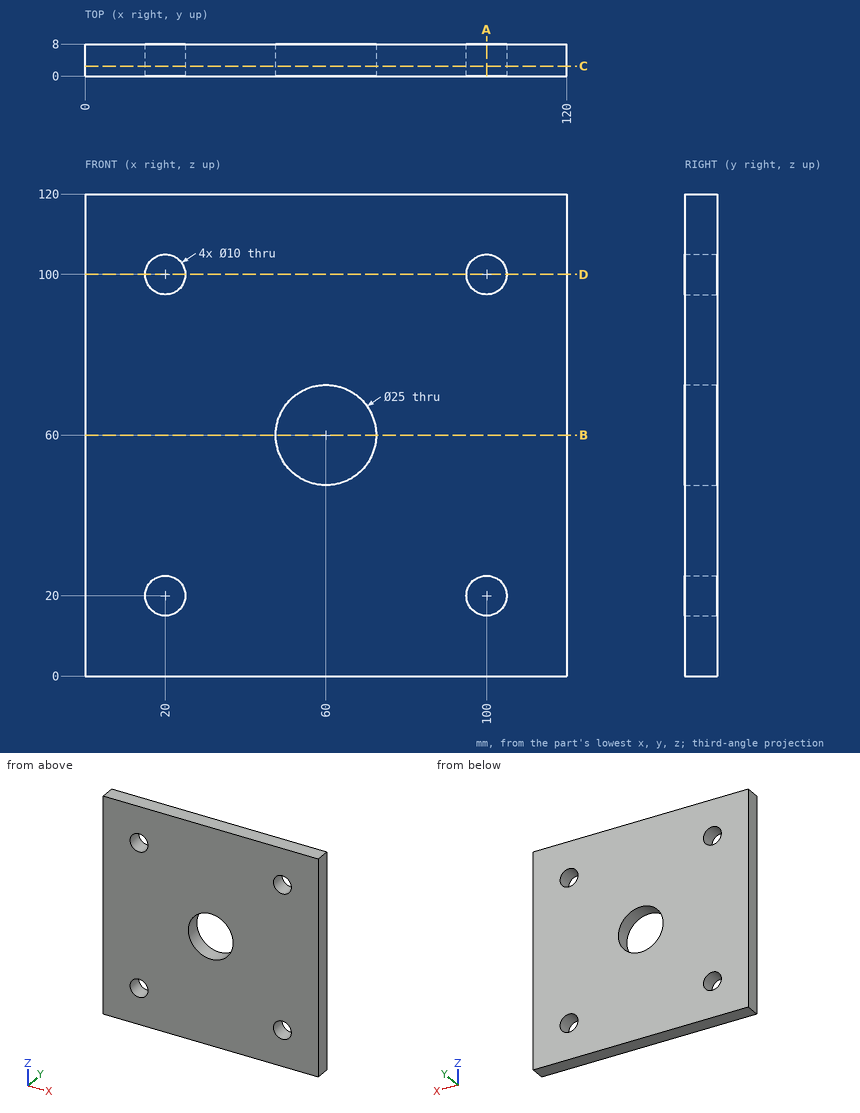
Part print with two shaded views. Sizes in mm from the minimum x, y, z corner. Coordinates: 2 decimals unless noted, no trailing zeros. Write each loop counter-clockwise with the first axis right and the second up, starting at its lowest first coordinate (ties: lowest second). Pieces come first, ordered by that corner, then holes.
1. Drop flat-ended pins along their axis: pin 1 (15 mm diameter, centred on x = 60, z = 60, fed in from +Y); pin 2 (8 mm diameter, centred on x = 33.5, z = 82.5, fed in from -Y). Give the stop position or say it passes through.
Answer block:
pin 1: passes through
pin 2: stops at y = 0
2. Band-saw the part on B-B, the plane z = 60. Give the cut face in (x, y), and give its area (3 significant figures).
Answer block:
outline: (0, 0) - (47.5, 0) - (47.5, 8) - (0, 8) - close; (72.5, 0) - (120, 0) - (120, 8) - (72.5, 8) - close
area: 760 mm2
3. Band-saw the part on C-C, the plane y = 2.5. Give the cut face in (x, z), and give its area (3 significant figures).
Answer block:
outline: (0, 0) - (120, 0) - (120, 120) - (0, 120) - close; hole circle Ø10 at (20, 20); hole circle Ø10 at (20, 100); hole circle Ø25 at (60, 60); hole circle Ø10 at (100, 20); hole circle Ø10 at (100, 100)
area: 13,600 mm2
4. Band-saw the part on A-A, the plane x = 100. Give the cut face in (y, z).
Answer block:
outline: (0, 0) - (8, 0) - (8, 15) - (0, 15) - close; (0, 25) - (8, 25) - (8, 95) - (0, 95) - close; (0, 105) - (8, 105) - (8, 120) - (0, 120) - close
5. Drill centre lines: probe 1 along Z at (x, y) = (20, 2.75); probe 2 along Z at (x, y) = (21, 1). Where is each one in solid material? Low to high.
Answer block:
probe 1: z = 0 to 15, 25 to 95, 105 to 120
probe 2: z = 0 to 15.1, 24.9 to 95.1, 104.9 to 120
6. Band-saw the part on D-D, the plane z = 100. Give the cut face in (x, y).
Answer block:
outline: (0, 0) - (15, 0) - (15, 8) - (0, 8) - close; (25, 0) - (95, 0) - (95, 8) - (25, 8) - close; (105, 0) - (120, 0) - (120, 8) - (105, 8) - close
